Autodesk Inventor part; units mm, degrees
ref_plane "작업 평면1" through (0, 0, 12.5) normal (0, 0, 1) x (1, 0, 0)
ref_plane "작업 평면2" through (0, 0, -12.5) normal (0, 0, 1) x (1, 0, 0)
ref_plane "작업 평면3" through (0, 0, 8) normal (0, 0, 1) x (1, 0, 0)
sketch "스케치1" plane through (0, 0, 0) normal (0, 1, 0) x (-1, 0, 0)
  line L0 (17.5, 0) -> (-17.5, 0)
  line L1 (0, -17.5) -> (0, 17.5)
  circle A0 centre (0, 0) radius 5.25
  circle A1 centre (0, 0) radius 12.5
  dimension "d0" = 10.5
  dimension "d1" = 25
extrude "돌출1" add sketch "스케치1" along normal blind 20 contours A1 L1 A0 L0 | L0 A0 L1 A1 | L1 A0 L0 A1 | A1 L0 A0 L1
ref_plane "작업 평면1" through (0, 0, 12.5) normal (0, 0, 1) x (1, 0, 0)
sketch "스케치2" plane through (0, 0, 12.5) normal (0, 0, 1) x (1, 0, 0)
  line L0 (0, 0) -> (0, 8)
  circle A0 centre (0, 8) radius 2
  dimension "d5" = 8
  dimension "d6" = 4
extrude "돌출2" cut sketch "스케치2" against normal blind 40
sketch "스케치3" plane through (0, 0, 12.5) normal (0, 0, 1) x (1, 0, 0)
  line L0 (0, 0) -> (0, 8)
  circle A0 centre (0, 8) radius 4
  point P0 (0, 6)
  point P1 (0, 10)
  dimension "d10" = 8
  dimension "d11" = 8
extrude "돌출3" cut sketch "스케치3" against normal blind 3
ref_plane "작업 평면2" through (0, 0, -12.5) normal (0, 0, 1) x (1, 0, 0)
sketch "스케치4" plane through (0, 0, -12.5) normal (0, 0, 1) x (1, 0, 0)
  line L0 (0, 0) -> (0, 8)
  circle A0 centre (0, 8) radius 2
  line L1 (0, 8) -> (-2.05, 4.4493)
  line L2 (0, 8) -> (2.05, 4.4493)
  line L3 (2.05, 4.4493) -> (-2.05, 4.4493)
  line L4 (4.1, 8) -> (2.05, 4.4493)
  line L5 (2.05, 11.5507) -> (4.1, 8)
  line L6 (-2.05, 11.5507) -> (2.05, 11.5507)
  line L7 (-4.1, 8) -> (-2.05, 11.5507)
  line L8 (-2.05, 4.4493) -> (-4.1, 8)
  point P0 (2.05, 4.4493)
  point P1 (4.1, 8)
  point P2 (2.05, 11.5507)
  point P3 (-2.05, 11.5507)
  point P4 (-4.1, 8)
  point P5 (-2.05, 4.4493)
  dimension "d15" = 8
  dimension "d16" = 4.1
  dimension "d17" = 30
  dimension "d20" = 360
extrude "돌출4" cut sketch "스케치4" along normal blind 4
fillet "모깎기1" radius 2 1 edges at (12.5, 20, 0)
sketch "스케치6" plane through (0, 0, 0) normal (0, 0, 1) x (1, 0, 0)
  line L0 (8, 32) -> (8, 22.5)
  line L1 (-15.1828, 0) -> (17.5971, 0)
  line L2 (0, -6.4) -> (0, 38.4)
  arc A0 (12.5, 18) -> (10.5, 20) centre (10.5, 18) ccw
  arc A1 (8, 22.5) -> (10.5, 20) centre (10.5, 22.5) ccw
  line L3 (-10.5, 20) -> (10.5, 20)
  line L4 (8, 32) -> (0, 32)
  point P0 (0, 0)
  point P1 (0, 20)
  dimension "d24" = 8
  dimension "d26" = 12
revolve "회전1" add sketch "스케치6" angle 360 about axis through (0, -10, 0) along (0, 1, 0)
ref_plane "작업 평면3" through (0, 0, 8) normal (0, 0, 1) x (1, 0, 0)
sketch "스케치8" plane through (0, 32, 0) normal (0, 1, 0) x (1, 0, 0)
  circle A0 centre (0, 0) radius 2.5
  line L0 (0, 3.5) -> (-0.4341, 2.462)
  line L1 (-0.4341, 2.462) -> (0, 3.5)
  line L2 (0, 17.5005) -> (0, -17.5027)
  line L3 (0.4341, 2.462) -> (0, 3.5)
  line L4 (-1.1971, 3.2889) -> (-1.25, 2.1651)
  line L5 (-0.4341, 2.462) -> (-1.1971, 3.2889)
  line L6 (-2.2498, 2.6812) -> (-1.9151, 1.607)
  line L7 (-1.25, 2.1651) -> (-2.2498, 2.6812)
  line L8 (-3.0311, 1.75) -> (-2.3492, 0.8551)
  line L9 (-1.9151, 1.607) -> (-3.0311, 1.75)
  line L10 (-3.4468, 0.6078) -> (-2.5, 0)
  line L11 (-2.3492, 0.8551) -> (-3.4468, 0.6078)
  line L12 (-3.4468, -0.6078) -> (-2.3492, -0.8551)
  line L13 (-2.5, 0) -> (-3.4468, -0.6078)
  line L14 (-3.0311, -1.75) -> (-1.9151, -1.607)
  line L15 (-2.3492, -0.8551) -> (-3.0311, -1.75)
  line L16 (-2.2498, -2.6812) -> (-1.25, -2.1651)
  line L17 (-1.9151, -1.607) -> (-2.2498, -2.6812)
  line L18 (-1.1971, -3.2889) -> (-0.4341, -2.462)
  line L19 (-1.25, -2.1651) -> (-1.1971, -3.2889)
  line L20 (0, -3.5) -> (0.4341, -2.462)
  line L21 (-0.4341, -2.462) -> (0, -3.5)
  line L22 (1.1971, 3.2889) -> (1.25, 2.1651)
  line L23 (0.4341, 2.462) -> (1.1971, 3.2889)
  line L24 (2.2498, 2.6812) -> (1.9151, 1.607)
  line L25 (1.25, 2.1651) -> (2.2498, 2.6812)
  line L26 (3.0311, 1.75) -> (2.3492, 0.8551)
  line L27 (1.9151, 1.607) -> (3.0311, 1.75)
  line L28 (3.4468, 0.6078) -> (2.5, 0)
  line L29 (2.3492, 0.8551) -> (3.4468, 0.6078)
  line L30 (3.4468, -0.6078) -> (2.3492, -0.8551)
  line L31 (2.5, 0) -> (3.4468, -0.6078)
  line L32 (3.0311, -1.75) -> (1.9151, -1.607)
  line L33 (2.3492, -0.8551) -> (3.0311, -1.75)
  line L34 (2.2498, -2.6812) -> (1.25, -2.1651)
  line L35 (1.9151, -1.607) -> (2.2498, -2.6812)
  line L36 (1.1971, -3.2889) -> (0.4341, -2.462)
  line L37 (1.25, -2.1651) -> (1.1971, -3.2889)
  line L38 (0, 2.5) -> (0, 3.5)
  point P0 (-2.5, 0)
  point P1 (2.5, 0)
  dimension "d33" = 5
  dimension "d36" = 180
  dimension "d38" = 1
extrude "돌출6" cut sketch "스케치8" against normal up to surface (12 mm away)
properties part number "가변저항-조향 연결"
Model file for the job. Use its own axes, mm. A direction names the side the tool comes from. Give positions to 0.01 mm unless a question says otherwise; leave off trailing zeros. Order: outer loops, then holes, each group sorted by start corner. A loop starts at its lowest first (then second) coordinate and runs counter-clockwise, first axis right, second up. Notation, with made-up numbers: (-6.5, 21) - (12.5, 21) arc R27 cw to (12.5, 56) - close; hole circle Ø4 at (75, 57.25). An arc over 180 degrees is marked (long way). Return JSON: item names as keys, results as strings.
1) Probe line 1 (Y direction, x = 0, z = 6.5); line 2 (X direction, y = 13.25, z = 0); line 3 (Z direction, x = -0.25, y = 13). List the from-to ranges inside material, lowest first. Write a range as from..to.
Geometry says:
{"line 1": "0..6, 10..32", "line 2": "-12.5..-5.25, 5.25..12.5", "line 3": "-12.5..-5.24, 5.24..12.5"}
2) Pull direction Z, two halves, no side cores. Call faces 3 (the flat face through (-2, 7, 9.5)), 4 (the flat face through (0, 11.551, -11)), 5 (the flat face through (0.81, 26.08, -2.87)), 6 (the flat face through (-2.48, 26.08, 1.68)): pulls with the +Z half, pulls with the -Z half, needs draft (parallel to the pull), parting line crosses it, or undercut.
Geometry says:
{"face 3": "pulls with the +Z half", "face 4": "needs draft", "face 5": "undercut", "face 6": "undercut"}
3) 3-axis set-ups, long thin cutter, end or side, ignore diameter. For faces 1 (the cylindrical face through (-11.547, 8.874, 4.788)), 2 (the cylindrical face through (-2.42, 9.86, 4.66)): which of +Z, -Z, +X, -X, +Y, -Y reach the whole face in a straight line?
Geometry says:
{"face 1": "+Y, -Y", "face 2": "-Y"}
4) Flat gauge pins, fed straight in: P1, Ø1, axis at x = -8, z = 6.5, coming from the +Y side; P2, Ø5, axis at x = -8, z = -10, coming from the +Y side; P3, Ø7, axis at x = 0, y = 8, coming from the +Z side. Where does each tip first touch, or does it go through?
Geometry says:
{"P1": "y = 20.1", "P2": "y = 20.01", "P3": "z = 9.5"}
5) Cut at A-A, the plane y = 19. Give the cut face in (x, z), plus the area to 3 significant figures.
Geometry says:
{"outline": "circle Ø24.46 at (0, 0); hole circle Ø10.5 at (0, 0)", "area": "383 mm²"}
